Can you work these out from the model? Positions are in its coordinate system, mm. A direction names the side the tool comes from. Give positions to 0.01 mm unless a question says otherwise; leave off trailing zeros. Loops run counter-clockwise (first coordinate to the right, second up) from the corner with the lowest first, then second, coordinate; pieces in that order, holes last. Notation, with made-up numbers: (36.25, 71) - (92.25, 71) arc R22 ccw to (92.25, 98) - close; hole circle Ø8 at (74, 77.5). An arc over 180 degrees is marked (long way). Answer as a JSON object with one key per item and string values. Group by question number.
Item 1: Suppose I cut it at B-B on y = 0. Write out the boundary of the cut face in (x, z) (3 decimals).
Item 2: Which directions (+Z, -Z, +X, -X, +Y, -Y) give clear straight access to the entire face, cutting with the end or side of a thin tool? Please do faces 1 (the flat face through (-38.1, 0, 0)), 2 (the flat face through (38.1, 0, 0)).
Item 3: Suppose I cut it at A-A on x = 23.5. Write out the boundary of the cut face in (y, z).
Item 4: Suppose I cut it at C-C on z = 0. Write out the boundary of the cut face in (x, y).
Item 5: Thinking about a two-plate mould opening in Z: for faces 3 (the cylindrical face through (38, -0.8, -44.5)), 4 (the flat face through (63.5, 0, -51)), 5 (the flat face through (0, 0, -101.6)), which applies, pulls with the +Z half, pulls with the -Z half, needs draft (parallel to the pull), parting line crosses it, or undercut?
Item 6: Suppose I cut it at D-D on x = 0. Write out the boundary of the cut face in (y, z) (3 decimals).
Item 7: Please list where these lines run through material, in increasing order: L1, parallel to X at y = 2.5, z = -9; L2, parallel to Z at x = 25.5, y = 4; L3, parallel to Z at x = 20, y = 1.
Item 8: Will these pins go through, and if not, where does the flat tip stop? pin 1 (11.5 mm diameter, centred on y = 2, z = 7, fed in from +X); pin 2 (6 mm diameter, centred on x = -21, z = -16, fed in from +Y); pin 3 (1 mm diameter, centred on x = 24, y = -12, fed in from +Z).
from build123d import *

# Parameters (mm, degrees)
F0_R     = 19.05
F1_DEPTH = 38.1
F2_R     = 14.605
F3_DEPTH = 101.6
F4_R     = 6.35
F5_DEPTH = 63.5


with BuildPart() as f1:
    # F0 (on Right) → F1 (new body, symmetric)
    with BuildSketch(Plane.YZ):
        Circle(F0_R)
    extrude(amount=F1_DEPTH, both=True)

    # F2 (on Top) → F3 (join)
    with BuildSketch(Plane.XY):
        Circle(F2_R)
    extrude(amount=-F3_DEPTH)

    # F4 (on Right) → F5 (join)
    with BuildSketch(Plane.YZ):
        with Locations((0, -50.8)):
            Circle(F4_R)
    extrude(amount=F5_DEPTH)


solid = f1.part
Worked out:
{
 "1": {"outline": "(-38.1, -19.05) - (-14.605, -19.05) - (-14.605, -101.6) - (14.605, -101.6) - (14.605, -57.15) - (63.5, -57.15) - (63.5, -44.45) - (14.605, -44.45) - (14.605, -19.05) - (38.1, -19.05) - (38.1, 19.05) - (-38.1, 19.05) - close"},
 "2": {"face 1": "+Z, -Z, -X, +Y, -Y", "face 2": "+Z, +X, +Y, -Y"},
 "3": {"outline": "circle Ø38.1 at (0, 0); circle Ø12.7 at (0, -50.8)"},
 "4": {"outline": "(-38.1, -19.05) - (38.1, -19.05) - (38.1, 19.05) - (-38.1, 19.05) - close"},
 "5": {"face 3": "undercut", "face 4": "needs draft", "face 5": "pulls with the -Z half"},
 "6": {"outline": "(-14.605, -101.6) - (14.605, -101.6) - (14.605, -12.231) arc R19.05 ccw (long way) to (-14.605, -12.231) - close"},
 "7": {"L1": "x = -38.1 to 38.1", "L2": "z = -55.73 to -45.87, -18.63 to 18.63", "L3": "z = -57.07 to -44.53, -19.02 to 19.02"},
 "8": {"pin 1": "stops at x = 38.1", "pin 2": "stops at y = 13.92", "pin 3": "stops at z = 15.19"}
}
